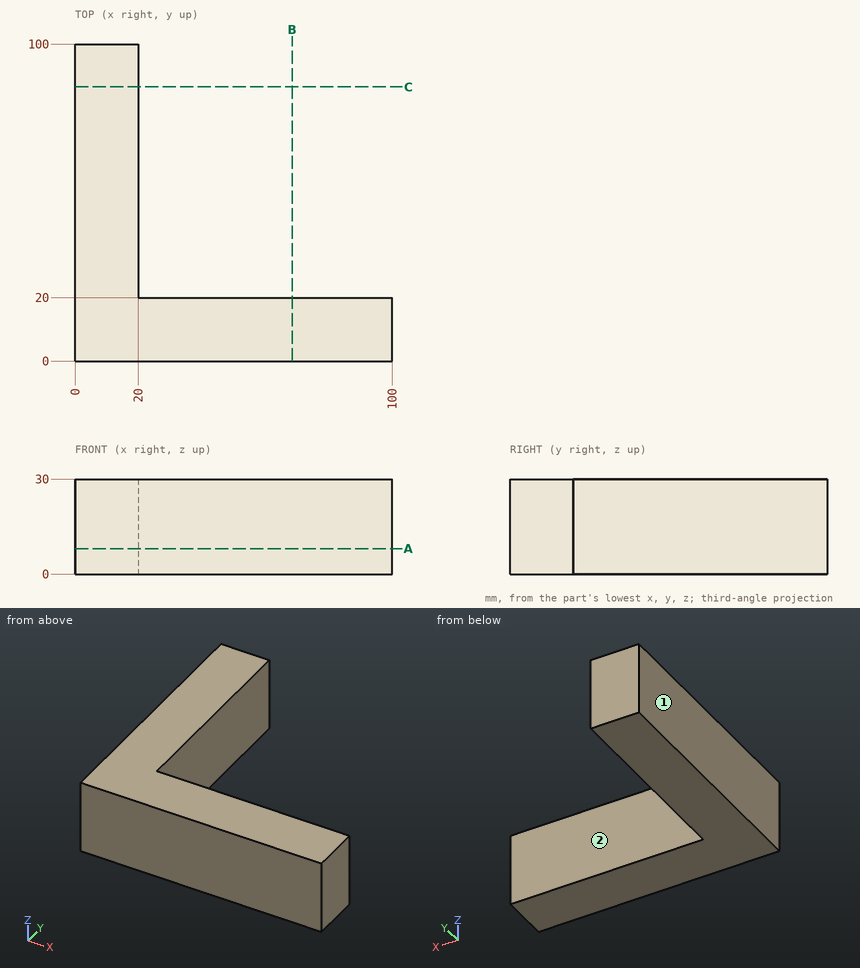
Geometry check sheet. Reference: drawing and pictorial views, mm from the part's lowest x, y, z. A direction names the side the tool comes from. Round coordinates to 2 decimals unless told otherwise and drop trailing zeros. Loops run counter-clockwise (first coordinate to the right, second up) from the corner with the lowest first, then second, coordinate; pieces in that order, holes last. Notation, with made-up numbers: (13, 49) - (27, 49) arc R29 cw to (27, 71) - close; hole circle Ø10 at (26, 7). An arc over 180 degrees is marked (long way). Use a Markdown table: item, result.
Q1. Material ranges on line 1 (X direction, y = 56, z = 20.5), recorded low to high.
Solutions:
| item | result |
|---|---|
| line 1 | x = 0 to 20 |
Q2. Access from +Z, -Z, +X, -X, +Y, -Y to the whole of each face (thin tool, end or side, straight path). Record for the marked faces 1 and 2.
Solutions:
| item | result |
|---|---|
| face 1 | +Z, -Z, -X, +Y, -Y |
| face 2 | +Z, -Z, +X, +Y |
Q3. Cross-section at A-A on z = 8. Record the cut outline in (x, y), plus the area to 3 significant figures.
Solutions:
| item | result |
|---|---|
| outline | (0, 0) - (100, 0) - (100, 20) - (20, 20) - (20, 100) - (0, 100) - close |
| area | 3,600 mm2 |
Q4. Go/stop test with flat-tipped pins: P1, Ø1.5, axis at y = 86, z = 26.5, coming from the +X side; P2, Ø3, axis at x = 61.5, z = 21.5, coming from the +Y side. Record where each tip stops, or that it passes through.
Solutions:
| item | result |
|---|---|
| P1 | stops at x = 20 |
| P2 | stops at y = 20 |
Q5. Cross-section at B-B on x = 68.5. Record the cut outline in (y, z), plus the area to 3 significant figures.
Solutions:
| item | result |
|---|---|
| outline | (0, 0) - (20, 0) - (20, 30) - (0, 30) - close |
| area | 600 mm2 |
